from build123d import *

# Parameters (mm, degrees)
CUT_EXTRUDE_2_DEPTH = 1.2
FILLET_1_R          = 0.1


with BuildPart() as part:
    # 草图8 → Revolve 1380 (revolve)
    with BuildSketch(Plane(origin=(0, 0, 0), x_dir=(0, 0, -1), z_dir=(1, 0, 0))):
        with BuildLine():
            Line((0, 0), (-14.4, 0))
            ThreePointArc((-14.4, 0), (-14.180811394, 1.464186604), (-13.542463035, 2.8))
            Line((-13.542463035, 2.8), (-12, 2.8))
            Line((-12, 2.8), (-12, 1.45))
            Line((-12, 1.45), (-2.511473671, 1.45))
            Line((-2.511473671, 1.45), (0, 0))
        make_face()
    revolve(axis=Axis((0, 0, 11.71), (0, 0, -1)))

    # 草图7 → 切除-拉伸2 (cut)
    with BuildSketch(Plane.XY.offset(14.4)):
        with BuildLine():
            Line((0.2, 0.928708781), (0.2, 0.797500009))
            ThreePointArc((0.2, 0.797500009), (0.375003701, 0.375003701), (0.797500009, 0.2))
            Line((0.797500009, 0.2), (0.928708781, 0.2))
            ThreePointArc((0.928708781, 0.2), (0.95, 0), (0.928708781, -0.2))
            Line((0.928708781, -0.2), (0.797500009, -0.2))
            ThreePointArc((0.797500009, -0.2), (0.375003701, -0.375003701), (0.2, -0.797500009))
            Line((0.2, -0.797500009), (0.2, -0.928708781))
            ThreePointArc((0.2, -0.928708781), (0, -0.95), (-0.2, -0.928708781))
            Line((-0.2, -0.928708781), (-0.2, -0.797500009))
            ThreePointArc((-0.2, -0.797500009), (-0.375003701, -0.375003701), (-0.797500009, -0.2))
            Line((-0.797500009, -0.2), (-0.928708781, -0.2))
            ThreePointArc((-0.928708781, -0.2), (-0.95, 0), (-0.928708781, 0.2))
            Line((-0.928708781, 0.2), (-0.797500009, 0.2))
            ThreePointArc((-0.797500009, 0.2), (-0.375003701, 0.375003701), (-0.2, 0.797500009))
            Line((-0.2, 0.797500009), (-0.2, 0.928708781))
            ThreePointArc((-0.2, 0.928708781), (0, 0.95), (0.2, 0.928708781))
        make_face()
    extrude(amount=-CUT_EXTRUDE_2_DEPTH, mode=Mode.SUBTRACT)

    # 圆角1
    fillet_1_edges = [part.edges().sort_by_distance(p)[0] for p in [
        (0, -1.45, 12),
    ]]
    fillet(fillet_1_edges, radius=FILLET_1_R)


solid = part.part
Check sheet for the modelled part. Datum: model origin and axes. Units: mm. Round coordinates to 2 decimals unless told otherwise and drop trailing zeros. Write each loop counter-clockwise with the first axis right and the second up, starting at its lowest first coordinate (ties: lowest second). Pieces come first, ordered by that corner, then holes. Notation, with made-up numbers: (-30.5, -34.75) -> (-6.5, -34.75) arc R17 ccw to (-6.5, -29.75) -> close; hole circle Ø11 at (1, 54.5). An arc over 180 degrees is marked (long way). Answer as CSV lines item,"result". Start each with the question number.
1) Go/stop test with flat-tipped pins: P1, Ø2, axis at x = 1, z = 3, coming from the -Y side; P2, Ø1.7, axis at x = 1.5, y = 0, coming from the -Z side; P3, Ø1, axis at x = 1.5, y = 1.5, coming from the -Z side; P4, Ø3, axis at x = 0.5, y = 1.5, coming from the +Z side. Record where each tip stops, or that it passes through.
2) Material ranges on line 1 (Y direction, x = 0.15, z = 12.5); line 2 (Z direction, x = 1.95, y = 1.35); line 3 (X direction, y = -2.55, z = 13.5), recorded low to high. Write a range as from..to.
3) Release check for a two-part mould opening along Y. For faces 1 (the flat face through (-1.21, 1.21, 12)), 2 (the cylindrical face through (0.1, -2.8, 12.8)), 3 (the flat face through (0, 0, 13.2)) record: pulls with the +Y half, pulls with the -Y half, needs draft (parallel to the pull), parting line crosses it, or undercut.
4) Section check B-B on y = -1.9. Enter the section's corners in (x, z), and give its area (3 significant figures).
5) Section check C-C on y = 2.2. Enter the section's corners in (x, z), and give its area (3 significant figures).
6) Section check A-A on z = 4.25. Enter the section's corners in (x, y).
7) Section check D-D on z = 1. Enter the section's corners in (x, y), and give its area (3 significant figures).
Found:
1,P1,"stops at y = -1.45"
1,P2,"stops at z = 1.13"
1,P3,"stops at z = 12"
1,P4,"stops at z = 14.37"
2,line 1,"y = -2.8..2.8"
2,line 2,"z = 12..13.8"
2,line 3,"x = -1.16..1.16"
3,face 1,"needs draft"
3,face 2,"parting line crosses it"
3,face 3,"undercut"
4,outline,"(-2.06, 12) -> (2.06, 12) -> (2.06, 13.54) arc R4.62 ccw to (-2.06, 13.54) -> close"
4,area,"7.68 mm^2"
5,outline,"(-1.73, 12) -> (1.73, 12) -> (1.73, 13.54) arc R4.49 ccw to (-1.73, 13.54) -> close"
5,area,"6.15 mm^2"
6,outline,"circle Ø2.9 at (0, 0)"
7,outline,"circle Ø1.15 at (0, 0)"
7,area,"1.05 mm^2"
